Input: part model. Units: mm. Frame: model coordinates. A direction names the side the tool comes from. Round coordinates to 2 decimals unless told otherwise and drop trailing zeros. Order: outer loops, then holes, each group sorted by start corner. A loop starts at its lowest first (then second) coordinate and runs counter-clockwise, first axis right, second up. Notation, with made-up numbers: (40, -23) -> (82, -23) arc R31 cw to (82, 16) -> close; hole circle Ø5 at (11, 57.25). An arc over 180 degrees is marked (long way). Use a Markdown table: item, result.
from build123d import *

# Parameters (mm, degrees)
BOSS_EXTRUDE1_DEPTH = 250
SKETCH2_R           = 1.5
CUT_EXTRUDE1_DEPTH  = 20
SKETCH3_R           = 1.5
CUT_EXTRUDE2_DEPTH  = 10


with BuildPart() as part:
    # Sketch1 → Boss-Extrude1 (new body)
    with BuildSketch(Plane.XY):
        Polygon((0, 0), (0, 17), (2, 17), (2, 2), (22, 2), (22, 0), align=None)
    extrude(amount=-BOSS_EXTRUDE1_DEPTH)

    # Sketch2 → Cut-Extrude1 (cut)
    with BuildSketch(Plane(origin=(0, 2, 0), x_dir=(1, 0, 0), z_dir=(0, 1, 0))):
        with Locations(Location((11, 226, 0), (0, 0, 270))):
            Circle(SKETCH2_R)
        with Locations(Location((11, 24, 0), (0, 0, 90))):
            Circle(SKETCH2_R)
        with Locations(Location((11, 125, 0), (0, 0, 270))):
            Circle(SKETCH2_R)
        with Locations(Location((11, 173, 0), (0, 0, 270))):
            Circle(SKETCH2_R)
        with Locations(Location((11, 77, 0), (0, 0, 270))):
            Circle(SKETCH2_R)
    extrude(amount=-CUT_EXTRUDE1_DEPTH, mode=Mode.SUBTRACT)

    # Sketch3 → Cut-Extrude2 (cut)
    with BuildSketch(Plane.ZY):
        with Locations((-207.5, 8.5)):
            Circle(SKETCH3_R)
        with Locations((-192.5, 8.5)):
            Circle(SKETCH3_R)
        with Locations((-67.5, 8.5)):
            Circle(SKETCH3_R)
        with Locations((-82.5, 8.5)):
            Circle(SKETCH3_R)
    extrude(amount=-CUT_EXTRUDE2_DEPTH, mode=Mode.SUBTRACT)


solid = part.part
1) Pin query (flat end, axial travel): pin 1 Ø10 at (y, z) = (9.5, -190.5) entering from +X; pin 2 Ø4 at (x, z) = (12.5, -53) entering from +Y. Return the tip coordinate at first contact, or that it passes through.
Results found:
| item | result |
|---|---|
| pin 1 | stops at x = 2 |
| pin 2 | stops at y = 2 |
2) Set-up query: faces 1 (the flat face through (2, 10, -123)), 2 (the flat face through (11, 0, -123)). Return all of +Z, -Z, +X, -X, +Y, -Y with unobstructed straight access to the full face (end or side cutting, diameter ignored); none if empty.
Results found:
| item | result |
|---|---|
| face 1 | +Z, -Z, +X, +Y |
| face 2 | +Z, -Z, +X, -X, -Y |
3) Line query: L1, parallel to X at y = 0.65, z = -24; L2, parallel to Z at x = 10.5, y = 1; L3, parallel to Y at x = 0.55, z = -67.5. Output: solid intervals per line, ascending. Write a range as [from, to].
Results found:
| item | result |
|---|---|
| L1 | x = [0, 9.5], [12.5, 22] |
| L2 | z = [-250, -227.41], [-224.59, -174.41], [-171.59, -126.41], [-123.59, -78.41], [-75.59, -25.41], [-22.59, 0] |
| L3 | y = [0, 7], [10, 17] |
4) Cut plane B-B on x = 19. Return loops of the section in (y, z), and give its area (3 significant figures).
Results found:
| item | result |
|---|---|
| outline | (0, -250) -> (2, -250) -> (2, 0) -> (0, 0) -> close |
| area | 500 mm² |
5) Cut plane A-A on z = -104. Return loops of the section in (x, y).
Results found:
| item | result |
|---|---|
| outline | (0, 0) -> (22, 0) -> (22, 2) -> (2, 2) -> (2, 17) -> (0, 17) -> close |
